```python
from build123d import *

# Parameters (mm, degrees)
SKETCH1_W           = 12.7
SKETCH1_H           = 80
BOSS_EXTRUDE1_DEPTH = 5.715


with BuildPart() as part:
    # Sketch1 → Boss-Extrude1 (new body)
    with BuildSketch(Plane(origin=(0, 0, 0), x_dir=(1, 0, 0), z_dir=(0, 1, 0))):
        Rectangle(SKETCH1_W, SKETCH1_H)
        Polygon((5, -40), (-5, -40), (-4.5, -45.715), (4.5, -45.715), align=None)
    extrude(amount=BOSS_EXTRUDE1_DEPTH)


solid = part.part
```
Geometry check sheet. Reference: the model listing, model coordinates, mm. A direction names the side the tool comes from. Round coordinates to 2 decimals unless told otherwise and drop trailing zeros. Order: outer loops, then holes, each group sorted by start corner. A loop starts at its lowest first (then second) coordinate and runs counter-clockwise, first axis right, second up. Notation, with made-up numbers: (-4, 47.25) - (39, 47.25) arc R33 ccw to (39, 81.25) - close; hole circle Ø8 at (0.5, 1.5). An arc over 180 degrees is marked (long way). Use a Markdown table: item, result. Add a question column.
(1) Tool access check on faces 1 (the flat face through (-6, 3, 40)), 2 (the flat face through (6, 3, 40)), 3 (the flat face through (0, 0, 2)). Record the directions out of +Z, -Z, +X, -X, +Y, -Y that give a thin tool (end or side, any length) a straight path to the whole face; none if there is none.
(2) Material ranges on line 1 along Z through (x, y) = (5.5, 3.9); line 2 along X through (y, z) = (3.3, 40.5), recorded low to high. Write a range as [from, to].
(3) Sectioned sample at A-A, the plane y = 3.85. Enter the section's corners in (x, z) (3 decimals), and give its area (3 significant figures).
(4) Depth check by flat-ended pin: pin 1 (0.7 mm diameter, centred on x = 5.5, y = 3, fed in from +Z). Enter the tip coordinate at first touch or a pass-through.
Answers below:
| question | item | result |
|---|---|---|
| 1 | face 1 | +Z, -X, +Y, -Y |
| 1 | face 2 | +Z, +X, +Y, -Y |
| 1 | face 3 | +Z, -Z, +X, -X, -Y |
| 2 | line 1 | [-40, 40] |
| 2 | line 2 | [-4.96, 4.96] |
| 3 | outline | (-6.35, -40) - (6.35, -40) - (6.35, 40) - (5, 40) - (4.5, 45.715) - (-4.5, 45.715) - (-5, 40) - (-6.35, 40) - close |
| 3 | area | 1,070 mm² |
| 4 | pin 1 | z = 40 |
